from build123d import *

# Parameters (mm, degrees)
SKETCH1_W           = 41.85
SKETCH1_H           = 10
SKETCH1_W_2         = 10
SKETCH1_H_2         = 29
BOSS_EXTRUDE1_DEPTH = 48
CUT_EXTRUDE1_DEPTH  = 48
SKETCH4_R           = 2
SKETCH4_R_2         = 4.2
CUT_EXTRUDE2_DEPTH  = 48
CUT_EXTRUDE3_DEPTH  = 48
SKETCH6_R           = 1
CUT_EXTRUDE4_DEPTH  = 2
SKETCH7_R           = 1
CUT_EXTRUDE5_DEPTH  = 1


with BuildPart() as part:
    # Sketch1 → Boss-Extrude1 (new body)
    with BuildSketch(Plane(origin=(0, 0, 0), x_dir=(1, 0, 0), z_dir=(0, 1, 0))):
        with Locations((-10.925, 5)):
            Rectangle(SKETCH1_W, SKETCH1_H)
        with Locations((5, -14.5)):
            Rectangle(SKETCH1_W_2, SKETCH1_H_2)
    extrude(amount=BOSS_EXTRUDE1_DEPTH)

    # Sketch3 → Cut-Extrude1 (cut)
    with BuildSketch(Plane(origin=(0, 48, 0), x_dir=(1, 0, 0), z_dir=(0, 1, 0))):
        Polygon((-31.85, 10), (-25.26317425, 10), (-31.85, 0), align=None)
    extrude(amount=-CUT_EXTRUDE1_DEPTH, mode=Mode.SUBTRACT)

    # Sketch4 → Cut-Extrude2 (cut)
    with BuildSketch(Plane.XY):
        with Locations((-5.589559388, 40.980827232)):
            Circle(SKETCH4_R)
        with Locations((-5.629681083, 24.979051073)):
            Circle(SKETCH4_R)
        with Locations((-21.591335547, 41.020948927)):
            Circle(SKETCH4_R)
        with Locations((-21.631457243, 25.019172768)):
            Circle(SKETCH4_R)
        with Locations((-13.629681083, 32.979051073)):
            Circle(SKETCH4_R_2)
    extrude(amount=-CUT_EXTRUDE2_DEPTH, mode=Mode.SUBTRACT)

    # Sketch5 → Cut-Extrude3 (cut)
    with BuildSketch(Plane(origin=(0, 48, 0), x_dir=(1, 0, 0), z_dir=(0, 1, 0))):
        Polygon((-25.26317425, 10), (10, 8), (10, 10), align=None)
    extrude(amount=-CUT_EXTRUDE3_DEPTH, mode=Mode.SUBTRACT)

    # Sketch6 → Cut-Extrude4 (cut)
    with BuildSketch(Plane(origin=(10, 0, 0), x_dir=(0, 0, -1), z_dir=(1, 0, 0))):
        with Locations((-21, 6.391948522)):
            Circle(SKETCH6_R)
        with Locations((-11, 15)):
            Circle(SKETCH6_R)
    extrude(amount=-CUT_EXTRUDE4_DEPTH, mode=Mode.SUBTRACT)

    # Sketch7 → Cut-Extrude5 (cut)
    with BuildSketch(Plane(origin=(0.484340621, 0, -8.539693864), x_dir=(-0.9983954953921488, 0, -0.056625389894163713), z_dir=(0.056625389894163713, 0, -0.9983954953921488))):
        with Locations((10.469048165, 7)):
            Circle(SKETCH7_R)
    extrude(amount=-CUT_EXTRUDE5_DEPTH, mode=Mode.SUBTRACT)


solid = part.part
Could you check a few things on this model? Use its own coordinates, in mm. A direction names the side the tool comes from. Give positions to 0.01 mm unless a question says otherwise; leave off trailing zeros. Loops run counter-clockwise (first coordinate to the right, second up) from the corner with the lowest first, then second, coordinate; pieces in that order, holes last. Notation, with made-up numbers: (-9, 86.5) -> (31, 86.5) arc R14 cw to (31, 92.5) -> close; hole circle Ø2 at (56, 80). An arc over 180 degrees is marked (long way). Return JSON: item names as keys, results as strings.
Item 1: I need wall thicknesses on L1, parallel to X at y = 39, z = 7.5; L2, parallel to X at y = 30, z = -6.5; L3, parallel to Y at x = 9, z = 11. Which ranges of each line are inside material? Lowest first, please. Write a range as from..to.
Geometry results:
{"L1": "x = 0..10", "L2": "x = -27.57..-16.59, -10.67..10", "L3": "y = 0..14, 16..48"}
Item 2: If we section it at D-D on y = 30: List the corners of the cut face in (x, z) for me.
Geometry results:
{"outline": "(-31.85, 0) -> (-25.26, -10) -> (-16.59, -9.51) -> (-16.59, 0) -> close; (-10.67, -9.17) -> (10, -8) -> (10, 29) -> (0, 29) -> (0, 0) -> (-10.67, 0) -> close"}
Item 3: Which directions (+Z, -Z, +X, -X, +Y, -Y) give clear straight access to the entire face, cutting with the end or side of a thin tool? Please do faces 4 (the flat face through (-16, 24, 0)), 5 (the flat face through (8, 15, 11)), 6 (the flat face through (-28.51, 24.34, -5.07)).
Geometry results:
{"face 4": "+Z, -X, +Y, -Y", "face 5": "+X", "face 6": "-Z, -X, +Y, -Y"}
Item 4: If we section it at A-A on y = 15: List the corners of the cut face in (x, z) for me, plus the area to 3 significant figures.
Geometry results:
{"outline": "(-31.85, 0) -> (-25.26, -10) -> (10, -8) -> (10, 10) -> (8, 10) -> (8, 12) -> (10, 12) -> (10, 29) -> (0, 29) -> (0, 0) -> close", "area": "636 mm²"}
Item 5: We'd pull the mould along Z, two halves only. Please class faces 1 (the cylindrical face through (-5.89, 26.962, -4.442)), 2 (the flat face through (-7.878, 24.336, -9.014)), 3 (the flat face through (8, 6, 21)): +Z half, -Z half, draft (parallel to the pull), parting line (faces both ways), or undercut.
Geometry results:
{"face 1": "draft", "face 2": "-Z half", "face 3": "undercut"}
Item 6: If we section it at C-C on z = 21: List the corners of the cut face in (x, y) for me.
Geometry results:
{"outline": "(0, 0) -> (10, 0) -> (10, 5.39) -> (8, 5.39) -> (8, 7.39) -> (10, 7.39) -> (10, 48) -> (0, 48) -> close"}
Item 7: I'm going to push flat-ended pins straight in: pin 1 (4.5 mm diameter, centred on x = -5.59, y = 40.98, fed in from -Z); pin 2 (6 mm diameter, centred on x = -25, y = 7, fed in from +Z); pin 3 (3.5 mm diameter, centred on x = -21.63, y = 25.02, fed in from +Z); pin 4 (1 mm diameter, centred on y = 6, z = 21, fed in from +X). Where does each tip first touch, or does it pass through?
Geometry results:
{"pin 1": "stops at z = -9.01", "pin 2": "stops at z = 0", "pin 3": "passes through", "pin 4": "stops at x = 8"}
Item 8: If we section it at B-B on x = -13: List the corners of the cut face in (y, z) for me.
Geometry results:
{"outline": "(0, -9.3) -> (28.83, -9.3) -> (28.83, 0) -> (0, 0) -> close; (37.13, -9.3) -> (48, -9.3) -> (48, 0) -> (37.13, 0) -> close"}
